from build123d import *

# Parameters (mm, degrees)
SKETCH_1_W              = 48
SKETCH_1_H              = 20
EXTRUDE_1_DEPTH         = 30
SKETCH_2_W              = 14
SKETCH_2_H              = 30
CUT_EXTRUDE_1_DEPTH     = 7
EXTRUDE_2_DEPTH         = 48
CUT_EXTRUDE_2_DEPTH     = 14
CUT_EXTRUDE_3_DEPTH     = 14
CUT_EXTRUDE_4_DEPTH     = 65.456478054
SKETCH_13_R             = 4
CUT_EXTRUDE_5_DEPTH     = 53.52066051
SKETCH_14_R             = 4
CUT_EXTRUDE_6_DEPTH     = 53.52066051
FILLET_1_R              = 7
EXTRUDE_5_DEPTH         = 1
SKETCH_20_R             = 7.5
CUT_EXTRUDE_8_DEPTH     = 53.52066051
BOSS_EXTRUDE1_DEPTH     = 25
CUT_EXTRUDE1_DEPTH      = 80.244164221
CUT_EXTRUDE1_DEPTH_BACK = 80.244164221


with BuildPart() as part:
    # Эскиз1 → Бобышка-Вытянуть1 (new body)
    with BuildSketch(Plane(origin=(0, 0, 0), x_dir=(1, 0, 0), z_dir=(0, 1, 0))):
        Rectangle(SKETCH_1_W, SKETCH_1_H)
    extrude(amount=EXTRUDE_1_DEPTH)

    # Эскиз2 → Вырез-Вытянуть1 (cut)
    with BuildSketch(Plane.XY.offset(10)):
        with Locations((0, 15)):
            Rectangle(SKETCH_2_W, SKETCH_2_H)
    extrude(amount=-CUT_EXTRUDE_1_DEPTH, mode=Mode.SUBTRACT)

    # Эскиз7 → Бобышка-Вытянуть2 (add)
    with BuildSketch(Plane(origin=(24, 0, 0), x_dir=(0, 0, -1), z_dir=(1, 0, 0))):
        Polygon((10, 0), (27.320508076, -10), (45.810889132, 22.026279442), (32, 30), (10, 30), align=None)
    extrude(amount=-EXTRUDE_2_DEPTH)

    # Эскиз8 → Вырез-Вытянуть2 (cut)
    with BuildSketch(Plane(origin=(24, 0, 0), x_dir=(0, 0, -1), z_dir=(1, 0, 0))):
        Polygon((10, 0), (10, 30), (32, 30), (45.810889132, 22.026279442), (27.320508076, -10), align=None)
    extrude(amount=-CUT_EXTRUDE_2_DEPTH, mode=Mode.SUBTRACT)

    # Эскиз9 → Вырез-Вытянуть3 (cut)
    with BuildSketch(Plane.ZY.offset(24)):
        Polygon((-10, 0), (-10, 30), (-32, 30), (-45.810889132, 22.026279442), (-27.320508076, -10), align=None)
    extrude(amount=-CUT_EXTRUDE_3_DEPTH, mode=Mode.SUBTRACT)

    # Эскиз11 → Вырез-Вытянуть4 (cut, through all)
    with BuildSketch(Plane.ZY.offset(10)):
        Polygon((-17.221869062, 5.518829477), (-27.321869062, 23.012542633), (-36.15532818, 17.912542633), (-26.05532818, 0.418829477), align=None)
    extrude(amount=-CUT_EXTRUDE_4_DEPTH, mode=Mode.SUBTRACT)

    # Эскиз13 → Вырез-Вытянуть5 (cut, through all)
    with BuildSketch(Plane(origin=(0, 0, -10), x_dir=(-1, 0, 0), z_dir=(0, 0, -1))):
        with Locations((17, 15)):
            Circle(SKETCH_13_R)
    extrude(amount=-CUT_EXTRUDE_5_DEPTH, mode=Mode.SUBTRACT)

    # Эскиз14 → Вырез-Вытянуть6 (cut, through all)
    with BuildSketch(Plane(origin=(0, 0, -10), x_dir=(-1, 0, 0), z_dir=(0, 0, -1))):
        with Locations((-17, 15)):
            Circle(SKETCH_14_R)
    extrude(amount=-CUT_EXTRUDE_6_DEPTH, mode=Mode.SUBTRACT)

    # Скругление1
    fillet_1_edges = [part.edges().sort_by_distance(p)[0] for p in [
        (-7, 15, 3),
        (7, 15, 3),
    ]]
    fillet(fillet_1_edges, radius=FILLET_1_R - 0.0001)  # a hair under: the kernel refuses the full size

    # Эскиз18 → Бобышка-Вытянуть5 (add)
    with BuildSketch(Plane(origin=(0, -14.330127019, -24.820508076), x_dir=(-1, 0, 0), z_dir=(0, -0.49999999999998845, -0.8660254037844453))):
        Polygon((2.153846154, 23.490381057), (2.153846154, 15.490381057), (1.025641026, 15.490381057), (1.025641026, 22.567304134), (-2.769230769, 22.567304134), (-2.769230769, 23.490381057), align=None)
    extrude(amount=EXTRUDE_5_DEPTH)

    # Эскиз20 → Вырез-Вытянуть8 (cut, through all)
    with BuildSketch(Plane(origin=(0, 0, -10), x_dir=(-1, 0, 0), z_dir=(0, 0, -1))):
        with Locations((-17, 15)):
            Circle(SKETCH_20_R)
        with Locations((17, 15)):
            Circle(SKETCH_20_R)
    extrude(amount=CUT_EXTRUDE_8_DEPTH, mode=Mode.SUBTRACT)

    # Sketch3 → Boss-Extrude1 (add)
    with BuildSketch(Plane(origin=(0, 30, 0), x_dir=(1, 0, 0), z_dir=(0, 1, 0))):
        with BuildLine():
            Line((7, -10), (24, -10))
            Line((24, -10), (24, 10))
            Line((24, 10), (10, 10))
            Line((10, 10), (10, 32))
            Line((10, 32), (-10, 32))
            Line((-10, 32), (-10, 10))
            Line((-10, 10), (-24, 10))
            Line((-24, 10), (-24, -10))
            Line((-24, -10), (-7, -10))
            ThreePointArc((-7, -10), (0, -3), (7, -10))
        make_face()
    extrude(amount=BOSS_EXTRUDE1_DEPTH)

    # Sketch4 → Cut-Extrude1 (cut, two sides: drawn at the far end of the back side and taken through both)
    with BuildSketch(Plane.ZY.offset(10).offset(-CUT_EXTRUDE1_DEPTH_BACK)):
        Polygon((-251.050138341, -96.468656337), (-45.810889132, 22.026279442), (35.63071017, 69.046608722), (240.869959379, 187.541544501), (3.880087821, 598.020042918), (-488.040009899, 314.00984208), align=None)
    extrude(amount=CUT_EXTRUDE1_DEPTH + CUT_EXTRUDE1_DEPTH_BACK, mode=Mode.SUBTRACT)


solid = part.part
Source: CAD feature listing. Evaluate the final solid. Frame: model axes, mm. A direction names the side the tool comes from. Coordinates: 2 decimals unless noted, no trailing zeros. Loops run counter-clockwise (first coordinate to the right, second up) from the corner with the lowest first, then second, coordinate; pieces in that order, holes last. Notation, with made-up numbers: (35, 9.25) - (93, 9.25) arc R16 cw to (93, 24.25) - close; hole circle Ø4 at (67, -35.5). An arc over 180 degrees is marked (long way). One line per question, with ' | ' between items.
1) Pull-direction query (X, two-part tool) for faces 5 (the face through (-2.154, 2, -35)), 6 (the face through (24, 27, 0)), 7 (the face through (0, 42, 3)); classes: released by +X, released by -X, zero draft, split by the parting line, or undercut.
Report:
face 5: released by -X | face 6: released by +X | face 7: undercut
2) Set-up query: faces 1 (the face through (-9.5, 15, -17)), 2 (the face through (-4.9, 15.2, 5)), 3 (the face through (10, 1, -22)), 4 (the face through (0, 0, 0)). Return all of +Z, -Z, +X, -X, +Y, -Y with unobstructed straight access to the full face (end or side cutting, diameter ignored); none if empty.
Report:
face 1: -Z, -X | face 2: +Z, +Y, -Y | face 3: -Z, +X, +Y, -Y | face 4: +Z, +X, -X, -Y
3) Line query: line 1 along Z through (x, y) = (-10.5, 28.5); line 2 along Z through (x, y) = (-6, 7). Output: solid intervals per line, ascending.
Report:
line 1: z = -10 to 10 | line 2: z = -37.14 to -29.85, -18.08 to 6.39
4) Section B-B, the plane z = 5.5. Give the number of separate pieces and of enclosed holes in the cut face, then the cut area to 3 significant figures.
Report:
separate pieces: 2 | enclosed holes: 2 | area: 1,820 mm²
5) Section C-C, the plane x = -8. Return loops of the section in (y, z).
Report:
outline: (-10, -27.32) - (22.03, -45.81) - (54.25, 10) - (0, 10) - (0, -10) - close; hole (0.42, -26.06) - (17.91, -36.16) - (23.01, -27.32) - (5.52, -17.22) - close
6) Section D-D, the plane z = -29.5. Return loops of the section in (x, y) (3 decimals).
Report:
outline: (-10, -6.225) - (10, -6.225) - (10, 6.385) - (-10, 6.385) - close; (-10, 21.755) - (10, 21.755) - (10, 31.443) - (-10, 31.443) - close
7) Section A-A, the plane x = 17. Return loops of the section in (y, z), then the cut area to 3 significant figures.
Report:
outline: (0, -10) - (11, -10) - (11, 10) - (0, 10) - close; (19, -10) - (42.7, -10) - (54.25, 10) - (19, 10) - close | area: 810 mm²
8) First-contact query: P1, Ø5, axis at x = 17, y = 15, coming from the -Z side; P2, Ø18, axis at y = 4.5, z = -24.5, coming from the -X side; P3, Ø12.5, axis at y = 27, z = -33.5, coming from the +X side; P4, Ø16, axis at x = 14.5, y = 14, coming from the -Z side. Flat tips, straight axial feed; report the tip coordinate or a pass-through.
Report:
P1: passes through | P2: stops at x = -10 | P3: stops at x = 10 | P4: stops at z = -45
